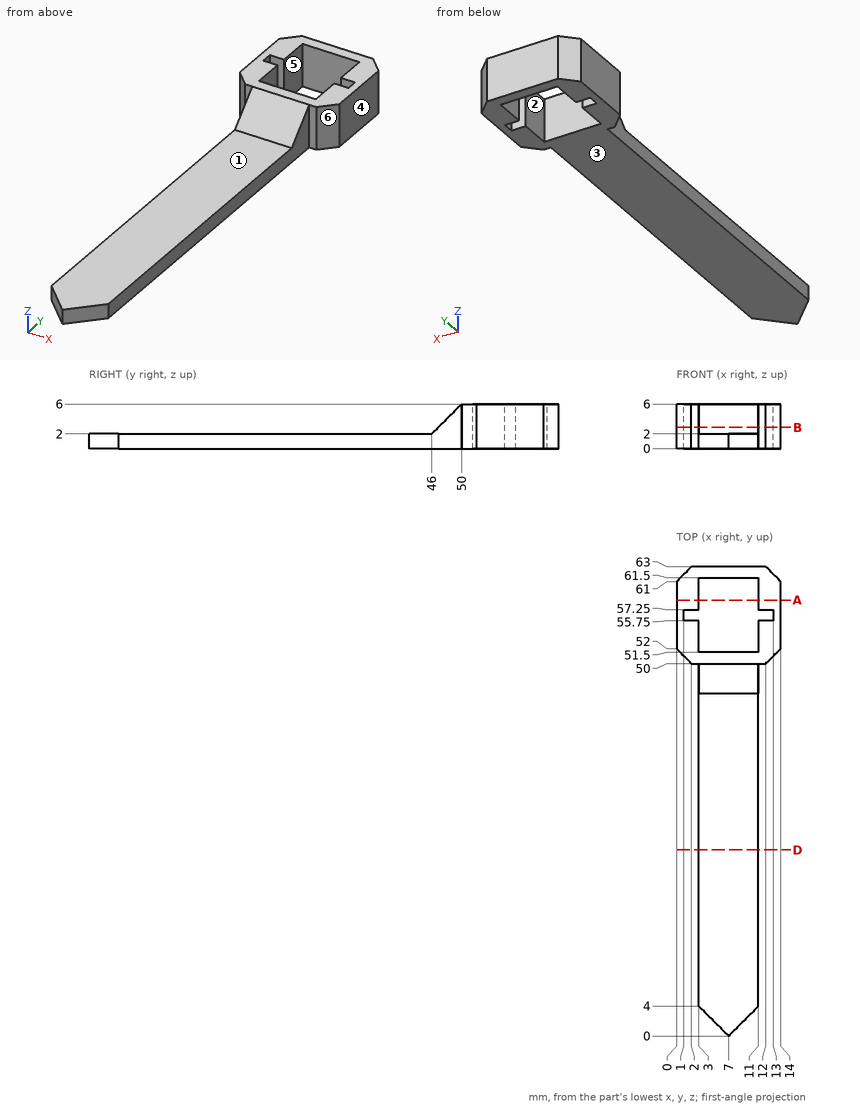
Here's the drawing with two shaded views (mm, measured from the low corner). I have some questions. A direction names the side the tool comes from. Coordinates: 2 decimals unless noted, no trailing zeros. Write each loop counter-clockwise with the first axis right and the second up, starting at its lowest first coordinate (ties: lowest second). Pieces come first, ordered by that corner, then holes. Notation, with made-up numbers: M 11,44 L 50,44 A13 cw 50,61 Z; hole C 68,17 d1. An arc over 180 degrees is marked long. Use one line per item in the form item = value.
Q1. For the marked faces 1, 2 and 3, which set-ups out of +Z, -Z, +X, -X, +Y, -Y let a thin tool reach every point of the face, with its end or its side?
Model answer:
face_1 = +Z, +X, -X, -Y
face_2 = +Z, -Z
face_3 = -Z, +X, -X, +Y, -Y
Q2. We'd pull the mould along Y, two halves only. Please class the marked faces 4, 5 and 6: +Y half, -Y half, draft (parallel to the pull), parting line (faces both ways), or undercut.
Model answer:
face_4 = draft
face_5 = undercut
face_6 = -Y half
Q3. For P1, Ø2.5, axis at x = 6, y = 32.5, coming from the +Z side; P2, Ø3, axis at x = 4, z = 4, coming from the -Y side; P3, Ø1, axis at x = 4, z = 5, coming from the -Y side; P4, Ø1.8, axis at y = 24, z = 4, coming from the +X side, each with a flat end and sliding along its axis, tell me the tip position at first contact or that it passes through.
Model answer:
P1 = 2
P2 = 46.5
P3 = 48.5
P4 = through
Q4. If we section it at D-D (y = 25): Write out the boundary of the cut face in (x, z).
Model answer:
outline = M 3,0 L 11,0 L 11,2 L 3,2 Z
Q5. If we section it at A-A (y = 58.5): Write out the boundary of the cut face in (x, z).
Model answer:
outline = M 0,0 L 3,0 L 3,6 L 0,6 Z; M 11,0 L 14,0 L 14,6 L 11,6 Z
Q6. I need wall thicknesses on line 1 along X through (y, z) = (58.5, 5); line 2 along Y through (x, z) = (2.75, 2.25); line 3 along Z through (x, y) = (6, 29.5). Which ranges of each line are inside material? Lowest first, please. Write a range as from..to.
Model answer:
line_1 = 0..3, 11..14
line_2 = 50..55.75, 57.25..63
line_3 = 0..2
Q7. If we section it at B-B (z = 2.85): Write out the boundary of the cut face in (x, y), then the cut area to 3 significant figures.
Model answer:
outline = M 0,52 L 2,50 L 3,50 L 3,46.85 L 11,46.85 L 11,50 L 12,50 L 14,52 L 14,61 L 12,63 L 2,63 L 0,61 Z; hole M 1,55.75 L 3,55.75 L 3,51.5 L 11,51.5 L 11,55.75 L 13,55.75 L 13,57.25 L 11,57.25 L 11,61.5 L 3,61.5 L 3,57.25 L 1,57.25 Z
area = 113 mm^2
